Autodesk Inventor part; units mm, degrees
ref_plane "YZ Plane" through (0, 0, 0) normal (1, 0, 0) x (0, 1, 0)
ref_plane "XZ Plane" through (0, 0, 0) normal (0, 1, 0) x (-1, 0, 0)
ref_plane "XY Plane" through (0, 0, 0) normal (0, 0, 1) x (1, 0, 0)
sketch "Sketch1" plane through (0, 0, 0) normal (0, 0, 1) x (1, 0, 0)
  line L0 (-3.6662, 6.35) -> (3.6662, 6.35)
  line L1 (3.6662, 6.35) -> (7.3323, 0)
  line L2 (7.3323, 0) -> (3.6662, -6.35)
  line L3 (3.6662, -6.35) -> (-3.6662, -6.35)
  line L4 (-3.6662, -6.35) -> (-7.3323, 0)
  line L5 (-7.3323, 0) -> (-3.6662, 6.35)
  circle A0 centre (0, 0) radius 6.858
  point P0 (2.5903, -6.35)
  point P1 (4.2041, -5.4183)
  point P2 (6.7944, -0.9317)
  point P3 (6.7944, 0.9317)
  point P4 (4.2041, 5.4183)
  point P5 (2.5903, 6.35)
  point P6 (-2.5903, 6.35)
  point P7 (-4.2041, 5.4183)
  point P8 (-6.7944, 0.9317)
  point P9 (-6.7944, -0.9317)
  point P10 (-4.2041, -5.4183)
  point P11 (-2.5903, -6.35)
  dimension "d0" = 12.7
  dimension "d1" = 13.716
extrude "Extrusion1" add sketch "Sketch1" along normal mid plane 32.639 contours L0 A0 L1 L2 L3 L4 L5
sketch "Sketch2" plane through (0, 0, 16.3195) normal (0, 0, 1) x (1, 0, 0)
  point P0 (0, 0)
hole "Hole1" at (0, 0, 16.3195) direction (0, 0, -1) diameter 3.683 end through all
mirror "Mirror1" about plane through (0, 0, 0) normal (0, 0, 1) of "Hole1"
properties part number "PINION_SHAFT_INTAKE" material "Aluminum, 7075-T6"
Part model, mm, in its own coordinate system. Coordinates: 2 decimals unless noted, no trailing zeros. Order: outer loops, then holes, each group sorted by start corner. A loop starts at its lowest first (then second) coordinate and runs counter-clockwise, first axis right, second up. Notation, with made-up numbers: (9.5, 35.25) - (36.5, 35.25) arc R29 cw to (36.5, 61.25) - close; hole circle Ø2 at (59.25, -32.5). An arc over 180 degrees is marked (long way). Return JSON: item names as keys, results as strings. Group by question number.
Item 1: Cut at A-A (y = 0). List the corners of the cut face in (x, z).
Item 2: Cut at C-C (z = 7). List the corners of the cut face in (x, y).
Item 3: Pull direction X, two halves, no side cores. Call faces 1 (the face through (1.634, -0.85, -0.228)), 2 (the face through (-5.52, 3.14, -0.23)), 3 (the face through (0, -6.35, 0)): pulls with the +X half, pulls with the -X half, needs draft (parallel to the pull), parting line crosses it, or undercut.
Item 4: Drill centre lines: probe 1 along Y at (x, z) = (0, -7); probe 2 along Y at (x, z) = (1, 13.5); probe 3 along X at (y, z) = (1.25, 11.5). Where is each one in solid material? Low to high. Write a range as from..to.
Item 5: Cut at B-B (x = 0). List the corners of the cut face in (y, z).
Item 6: Pin check, flat tips, straight feed: pin 1 (5 mm diameter, centred on y = -4, z = -9.5, fed in from +X); pin 2 (1.5 mm diameter, centred on x = 3.5, z = 1.5, fed in from +Y). Stop position of each tip, or through.
Item 7: Cut at D-D (y = -3.75). List the corners of the cut face in (x, z).
Check values:
{
 "1": {"outline": "(-6.86, -16.32) - (-1.84, -16.32) - (-1.84, 16.32) - (-6.86, 16.32) - close; (1.84, -16.32) - (6.86, -16.32) - (6.86, 16.32) - (1.84, 16.32) - close"},
 "2": {"outline": "(-6.79, -0.93) - (-4.2, -5.42) arc R6.86 ccw to (-2.59, -6.35) - (2.59, -6.35) arc R6.86 ccw to (4.2, -5.42) - (6.79, -0.93) arc R6.86 ccw to (6.79, 0.93) - (4.2, 5.42) arc R6.86 ccw to (2.59, 6.35) - (-2.59, 6.35) arc R6.86 ccw to (-4.2, 5.42) - (-6.79, 0.93) arc R6.86 ccw to start; hole circle Ø3.68 at (0, 0)"},
 "3": {"face 1": "undercut", "face 2": "pulls with the -X half", "face 3": "needs draft"},
 "4": {"probe 1": "y = -6.35..-1.84, 1.84..6.35", "probe 2": "y = -6.35..-1.55, 1.55..6.35", "probe 3": "x = -6.61..-1.35, 1.35..6.61"},
 "5": {"outline": "(-6.35, -16.32) - (-1.84, -16.32) - (-1.84, 16.32) - (-6.35, 16.32) - close; (1.84, -16.32) - (6.35, -16.32) - (6.35, 16.32) - (1.84, 16.32) - close"},
 "6": {"pin 1": "stops at x = 6.47", "pin 2": "stops at y = 6.28"},
 "7": {"outline": "(-5.17, -16.32) - (5.17, -16.32) - (5.17, 16.32) - (-5.17, 16.32) - close"}
}
